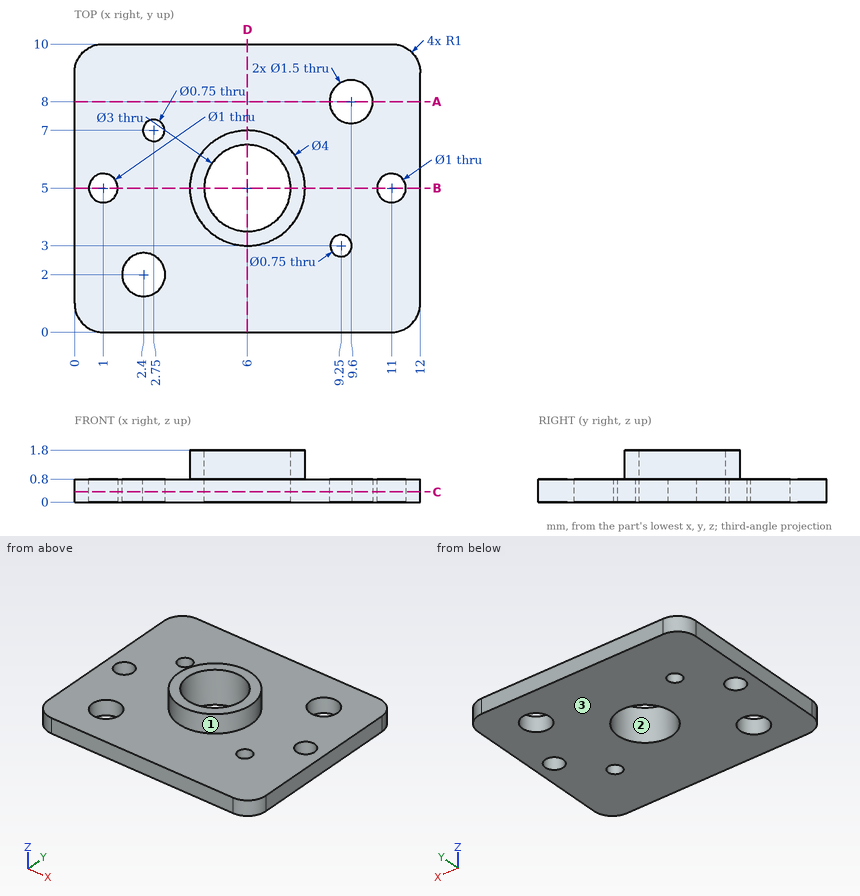
Check sheet for the drawn part. Datum: minimum x, y, z corner. Units: mm. Give positions to 0.01 mm unless a question says otherwise; leave off trailing zeros. Order: outer loops, then holes, each group sorted by start corner. A loop starts at its lowest first (then second) coordinate and runs counter-clockwise, first axis right, second up. Notation, with made-up numbers: (46.25, 45) -> (92.25, 45) arc R27 ccw to (92.25, 79) -> close; hole circle Ø9 at (71.25, -39). An arc over 180 degrees is marked (long way). Return JSON: item names as keys, results as strings.
1. Mould release check, pull along Y, two halves, no side actions. Record for the marked faces 1, 2 and 3: +Y half, -Y half, draft (parallel to the pull), parting line (faces both ways), or undercut.
From the geometry:
{"face 1": "parting line", "face 2": "undercut", "face 3": "draft"}
2. Cross-section at D-D, the plane x = 6. Record the cut outline in (y, z).
From the geometry:
{"outline": "(0, 0) -> (3.5, 0) -> (3.5, 1.8) -> (3, 1.8) -> (3, 0.8) -> (0, 0.8) -> close; (6.5, 0) -> (10, 0) -> (10, 0.8) -> (7, 0.8) -> (7, 1.8) -> (6.5, 1.8) -> close"}
3. Cross-section at A-A, the plane y = 8. Record the cut outline in (x, z).
From the geometry:
{"outline": "(0, 0) -> (8.85, 0) -> (8.85, 0.8) -> (0, 0.8) -> close; (10.35, 0) -> (12, 0) -> (12, 0.8) -> (10.35, 0.8) -> close"}
4. Go/stop test with a flat-tipped pin: P1, Ø1.2, axis at x = 9.6, y = 8, coming from the -Z side. Record where the tip stops, or that it passes through.
From the geometry:
{"P1": "through"}
5. Cross-section at B-B, the plane y = 5. Record the cut outline in (x, z).
From the geometry:
{"outline": "(0, 0) -> (0.5, 0) -> (0.5, 0.8) -> (0, 0.8) -> close; (1.5, 0) -> (4.5, 0) -> (4.5, 1.8) -> (4, 1.8) -> (4, 0.8) -> (1.5, 0.8) -> close; (7.5, 0) -> (10.5, 0) -> (10.5, 0.8) -> (8, 0.8) -> (8, 1.8) -> (7.5, 1.8) -> close; (11.5, 0) -> (12, 0) -> (12, 0.8) -> (11.5, 0.8) -> close"}
6. Cross-section at C-C, the plane z = 0.35. Record the cut outline in (x, y) (3 decimals).
From the geometry:
{"outline": "(0, 1) arc R1 ccw to (1, 0) -> (11, 0) arc R1 ccw to (12, 1) -> (12, 9) arc R1 ccw to (11, 10) -> (1, 10) arc R1 ccw to (0, 9) -> close; hole circle Ø1 at (1, 5); hole circle Ø1.5 at (2.4, 2); hole circle Ø0.75 at (2.75, 7); hole circle Ø3 at (6, 5); hole circle Ø1.5 at (9.6, 8); hole circle Ø0.75 at (9.25, 3); hole circle Ø1 at (11, 5)"}
7. Material ranges on probe 1 along Y at (x, z) = (11, 0.5); probe 2 along Y at (x, z) = (9.25, 0.45) (3 decimals); probe 3 along Z at (x, y) = (4, 9), recorded low to high. Write a range as [from, to].
From the geometry:
{"probe 1": "[0, 4.5], [5.5, 10]", "probe 2": "[0, 2.625], [3.375, 7.337], [8.663, 10]", "probe 3": "[0, 0.8]"}
